```python
from build123d import *

# Parameters (mm, degrees)
BOSS_EXTRUDE1_DEPTH = 58
SKETCH2_R           = 2.5
SKETCH2_R_2         = 20
CUT_EXTRUDE1_DEPTH  = 58
CUT_EXTRUDE2_DEPTH  = 58
CUT_EXTRUDE3_DEPTH  = 58
SKETCH5_R           = 2.95
BOSS_EXTRUDE2_DEPTH = 8
SKETCH7_W           = 29
SKETCH7_H           = 6
CUT_EXTRUDE5_DEPTH  = 10
SKETCH25_R          = 4
CUT_EXTRUDE6_DEPTH  = 10
SKETCH26_W          = 103.5
SKETCH26_H          = 2
CUT_EXTRUDE7_DEPTH  = 90
SKETCH29_R          = 1.5
CUT_EXTRUDE8_DEPTH  = 10


with BuildPart() as part:
    # Sketch1 → Boss-Extrude1 (new body)
    with BuildSketch(Plane(origin=(0, 0, 0), x_dir=(0, 0, -1), z_dir=(1, 0, 0))):
        Polygon((-73.351671883, 30.400809615), (-73.351671883, -29.599190385), (30.148328117, -29.599190385), (30.148328117, 30.400809615), (33.148328117, 30.400809615), (33.148328117, -34.599190385), (-76.351671883, -34.599190385), (-76.351671883, 30.400809615), align=None)
    extrude(amount=BOSS_EXTRUDE1_DEPTH)

    # Sketch2 → Cut-Extrude1 (cut)
    with BuildSketch(Plane.XY.offset(76.351671883)):
        with Locations((5.5, 24.900809615)):
            Circle(SKETCH2_R)
        with Locations((52.5, 24.900809615)):
            Circle(SKETCH2_R)
        with Locations((52.5, -22.099190385)):
            Circle(SKETCH2_R)
        with Locations((5.5, -22.099190385)):
            Circle(SKETCH2_R)
        with Locations((29, 1.400809615)):
            Circle(SKETCH2_R_2)
    extrude(amount=-CUT_EXTRUDE1_DEPTH, mode=Mode.SUBTRACT)

    # Sketch3 → Cut-Extrude2 (cut)
    with BuildSketch(Plane(origin=(0, 0, -33.148328117), x_dir=(-1, 0, 0), z_dir=(0, 0, -1))):
        with BuildLine():
            Line((-29, 30.400809615), (-58, 30.400809615))
            Line((-58, 30.400809615), (-58, 1.400809615))
            ThreePointArc((-58, 1.400809615), (-49.506096654, 21.90690627), (-29, 30.400809615))
        make_face()
    extrude(amount=-CUT_EXTRUDE2_DEPTH, mode=Mode.SUBTRACT)

    # Sketch4 → Cut-Extrude3 (cut)
    with BuildSketch(Plane(origin=(0, 0, -33.148328117), x_dir=(-1, 0, 0), z_dir=(0, 0, -1))):
        with BuildLine():
            Line((-29, 30.400809615), (0, 30.400809615))
            Line((0, 30.400809615), (0, 1.400809615))
            ThreePointArc((0, 1.400809615), (-8.493903346, 21.90690627), (-29, 30.400809615))
        make_face()
    extrude(amount=-CUT_EXTRUDE3_DEPTH, mode=Mode.SUBTRACT)

    # Sketch5 → Boss-Extrude2 (add)
    with BuildSketch(Plane(origin=(0, 0, -33.148328117), x_dir=(-1, 0, 0), z_dir=(0, 0, -1))):
        with Locations((-29, 1.400809615)):
            Circle(SKETCH5_R)
    extrude(amount=BOSS_EXTRUDE2_DEPTH)

    # Sketch7 → Cut-Extrude5 (cut)
    with BuildSketch(Plane.XY.offset(76.351671883)):
        with Locations((14.5, 1.400809615)):
            Rectangle(SKETCH7_W, SKETCH7_H)
    extrude(amount=-CUT_EXTRUDE5_DEPTH, mode=Mode.SUBTRACT)

    # Sketch25 → Cut-Extrude6 (cut)
    with BuildSketch(Plane.XZ.offset(34.599190385)):
        with Locations((29, 20.601671883)):
            Circle(SKETCH25_R)
    extrude(amount=-CUT_EXTRUDE6_DEPTH, mode=Mode.SUBTRACT)

    # Sketch26 → Cut-Extrude7 (cut)
    with BuildSketch(Plane(origin=(58, 0, 0), x_dir=(0, 0, -1), z_dir=(1, 0, 0))):
        with Locations((-21.601671883, -30.599190385)):
            Rectangle(SKETCH26_W, SKETCH26_H)
    extrude(amount=-CUT_EXTRUDE7_DEPTH, mode=Mode.SUBTRACT)

    # Sketch29 → Cut-Extrude8 (cut)
    with BuildSketch(Plane(origin=(0, -31.599190385, 0), x_dir=(1, 0, 0), z_dir=(0, 1, 0))):
        with Locations((19.5, -20.601671883)):
            Circle(SKETCH29_R)
        with Locations((24.25, -12.374430547)):
            Circle(SKETCH29_R)
        with Locations((33.75, -12.374430547)):
            Circle(SKETCH29_R)
        with Locations((38.5, -20.601671883)):
            Circle(SKETCH29_R)
        with Locations((33.75, -28.828913219)):
            Circle(SKETCH29_R)
        with Locations((24.25, -28.828913219)):
            Circle(SKETCH29_R)
    extrude(amount=-CUT_EXTRUDE8_DEPTH, mode=Mode.SUBTRACT)


solid = part.part
```
Source: CAD feature listing. Evaluate the final solid. Frame: model axes, mm. A direction names the side the tool comes from. Coordinates: 2 decimals unless noted, no trailing zeros. Loops run counter-clockwise (first coordinate to the right, second up) from the corner with the lowest first, then second, coordinate; pieces in that order, holes last. Notation, with made-up numbers: M 85,31.5 L 126,31.5 A38 cw 126,69.5 Z; hole C 48.25,-20.5 d1. An arc over 180 degrees is marked long. Use a Markdown table: item, result. Add a question column.
Q1. First-contact query: pin 1 (3 mm diameter, centred on x = 5.5, y = -22.1, fed in from +Z); pin 2 (17.5 mm diameter, centred on x = 38, y = -12, fed in from -Z); pin 3 (12 mm diameter, centred on x = 44, z = 20, fed in from +Y). Flat tips, straight axial feed; report the tip coordinate or a pass-through.
Q2. Section query C-C, the plane x = 45. Return loops of the section in (y, z).
Q3. Draft query along Y for faces 4 (the flat face through (36, -31.599, 22)), 5 (the flat face through (5, 4.401, 75)), 6 (the flat face through (22, -34.599, 21)), 7 (the cylindrical face through (37, -33.08, 20.54)). Return one class per face: pulls with the +Y half, pulls with the -Y half, needs draft (parallel to the pull), parting line crosses it, or undercut.
Q4. Section query D-D, the plane z = 56.5. Return loops of the section in (x, y), and give its area (3 significant figures).
Q5. Section query A-A, the plane x = 19.5. Return loops of the section in (y, z).
Q6. Access query for faces 1 (the flat face through (0, 18, 75)), 2 (the flat face through (16, -14, 73.352)), 3 (the cylindrical face through (48.982, 0.564, 74.873)). Directions: +Z, -Z, +X, -X, +Y, -Y. A direction counts if a zero-diameter tool reaches every point of the face in a straight line with its end or side. Return the directions, or none.
Q7. Section query B-B, the plane y = -5.5. Return loops of the section in (x, z), and give its area (3 significant figures).
Q8. Material intervals for L1, parallel to Y at x = 52.5, z = 74.6; L2, parallel to Z at x = 33.75, y = -32.7; L3, parallel to Y at x = 5.5, z = 74.1, sorted ascending.
Result:
| question | item | result |
|---|---|---|
| 1 | pin 1 | stops at z = -30.15 |
| 1 | pin 2 | stops at z = -33.15 |
| 1 | pin 3 | stops at y = -31.6 |
| 2 | outline | M -34.6,-33.15 L 25.59,-33.15 L 25.59,-30.15 L -31.6,-30.15 L -31.6,73.35 L -10.6,73.35 L -10.6,76.35 L -34.6,76.35 Z; M 13.4,73.35 L 30.4,73.35 L 30.4,76.35 L 13.4,76.35 Z |
| 3 | face 4 | pulls with the +Y half |
| 3 | face 5 | undercut |
| 3 | face 6 | pulls with the -Y half |
| 3 | face 7 | needs draft |
| 4 | outline | M 0,-34.6 L 58,-34.6 L 58,-31.6 L 0,-31.6 Z |
| 4 | area | 174 mm2 |
| 5 | outline | M -34.6,-33.15 L 28.8,-33.15 L 28.8,-30.15 L -31.6,-30.15 L -31.6,19.1 L -34.6,19.1 Z; M -34.6,22.1 L -31.6,22.1 L -31.6,73.35 L -16.2,73.35 L -16.2,76.35 L -34.6,76.35 Z; M 19,73.35 L 30.4,73.35 L 30.4,76.35 L 19,76.35 Z |
| 6 | face 1 | +Z, -Z, -X, +Y, -Y |
| 6 | face 2 | +X, -X, +Y |
| 6 | face 3 | +Z |
| 7 | outline | M 0,-33.15 L 58,-33.15 L 58,-30.15 L 0,-30.15 Z; M 0,73.35 L 10.23,73.35 L 10.23,76.35 L 0,76.35 Z; M 47.77,73.35 L 58,73.35 L 58,76.35 L 47.77,76.35 Z |
| 7 | area | 235 mm2 |
| 8 | L1 | y = -34.6 to -24.6, -19.6 to 22.4, 27.4 to 30.4 |
| 8 | L2 | z = -33.15 to 10.87, 13.87 to 27.33, 30.33 to 76.35 |
| 8 | L3 | y = -34.6 to -24.6, -19.6 to -1.6, 4.4 to 22.4, 27.4 to 30.4 |
